from build123d import *

# Parameters (mm, degrees)
F0_W     = 45
F0_H     = 10
F0_R     = 3
F0_R_2   = 2
F1_DEPTH = 10
F2_R     = 4
F3_R     = 3
F5_DEPTH = 2


with BuildPart() as f1:
    # F0 (on Top) → F1 (new body)
    with BuildSketch(Plane.XY):
        Rectangle(F0_W, F0_H)
        Circle(F0_R, mode=Mode.SUBTRACT)
        Circle(F0_R)
        Circle(F0_R_2, mode=Mode.SUBTRACT)
    extrude(amount=F1_DEPTH)

    # F2
    f2_edges = [f1.edges().sort_by_distance(p)[0] for p in [
        (-22.5, -5, 5),
        (22.5, -5, 5),
        (22.5, 5, 5),
        (-22.5, 5, 5),
    ]]
    fillet(f2_edges, radius=F2_R)

    # F3
    f3_edges = [f1.edges().sort_by_distance(p)[0] for p in [
        (0, -5, 10),
        (0, 5, 10),
        (21.328427, 3.828427, 10),
        (-21.328427, 3.828427, 10),
        (22.5, 0, 10),
        (-22.5, 0, 10),
        (21.328427, -3.828427, 10),
        (-21.328427, -3.828427, 10),
    ]]
    fillet(f3_edges, radius=F3_R)

    # F4 (on face) → F5 (cut)
    with BuildSketch(Plane.XY.offset(10)):
        with BuildLine():
            ThreePointArc((0, 2), (1.4142135624, 1.4142135624), (2, 0))
            ThreePointArc((2, 0), (1.4142135624, -1.4142135624), (0, -2))
            Line((0, -2), (2.2360679775, -2))
            ThreePointArc((2.2360679775, -2), (2.8025170769, -1.0704662693), (3, 0))
            ThreePointArc((3, 0), (2.8025170769, 1.0704662693), (2.2360679775, 2))
            Line((2.2360679775, 2), (0, 2))
        make_face()
        with BuildLine():
            Line((-2.2360679775, 2), (0, 2))
            Line((0, 2), (2.2360679775, 2))
            ThreePointArc((2.2360679775, 2), (0, 3), (-2.2360679775, 2))
        make_face()
        with BuildLine():
            ThreePointArc((0, -2), (-2, 0), (0, 2))
            Line((0, 2), (-2.2360679775, 2))
            ThreePointArc((-2.2360679775, 2), (-3, 0), (-2.2360679775, -2))
            Line((-2.2360679775, -2), (0, -2))
        make_face()
        with BuildLine():
            Line((2.2360679775, -2), (0, -2))
            Line((0, -2), (-2.2360679775, -2))
            ThreePointArc((-2.2360679775, -2), (0, -3), (2.2360679775, -2))
        make_face()
    extrude(amount=-F5_DEPTH, mode=Mode.SUBTRACT)


solid = f1.part
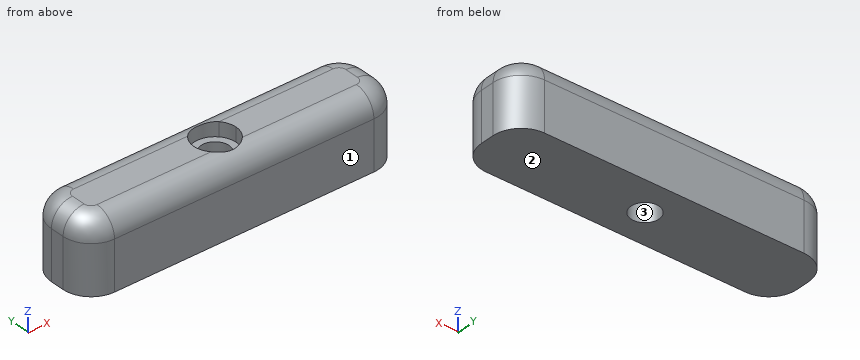
The listing builds one solid part. Answer for the finished solid, in the listing's coordinates (mm). Face numbers are marked on the shaded views. Coordinates: 2 decimals unless noted, no trailing zeros. Write each loop counter-clockwise with the first axis right and the second up, starting at its lowest first coordinate (ties: lowest second). Pieces come first, ordered by that corner, then holes. Notation, with made-up numbers: M -19.75,58 L 11.25,58 A17 cw 11.25,72 Z; hole C 11,10.5 d3. An arc over 180 degrees is marked long. Put each result on its own line as item: value. Start each with the question number.
1. A cutting plane is placed at A-A on z = 5.75. Write down the section's boundary in (x, y).
2. Consider line 1 (Y direction, x = 0, z = 4.75); line 2 (X direction, y = 0, z = 6); line 3 (X direction, y = 0, z = 8.65). Determine where each line is inside the solid, lowest interval first. Write a range as from..to.
3. A cutting plane is placed at B-B on x = 0. Write down the section's boundary in (y, z).
4. For a pull along Y with two mould halves and no side action, classify the marked faces 1, 2 and 3 as pulls with the +Y half, pulls with the -Y half, needs draft (parallel to the pull), parting line crosses it, or undercut.
5. A flat-ended cylindrical pin translates along its axis: P1, Ø3, axis at x = -0.5, y = -1, coming from the +Z side. Find the tip coordinate at first contact, or state that the pin passes through.
6. A cutting plane is placed at C-C on x = -8. Write down the section's boundary in (y, z), then the cut area to 3 significant figures.
Resolved:
1. outline: M -22.5,-1 A4 ccw -18.5,-5 L 18.5,-5 A4 ccw 22.5,-1 L 22.5,1 A4 ccw 18.5,5 L -18.5,5 A4 ccw -22.5,1 Z; hole C 0,0 d4
2. line 1: y = -5..-2, 2..5
2. line 2: x = -22.5..-2, 2..22.5
2. line 3: x = -22.01..-3, 3..22.01
3. outline: M -5,0 L -2,0 L -2,8 L -3,8 L -3,9.83 A3 ccw -5,7 Z; M 2,0 L 5,0 L 5,7 A3 ccw 3,9.83 L 3,8 L 2,8 Z
4. face 1: pulls with the -Y half
4. face 2: needs draft
4. face 3: undercut
5. P1: stops at z = 8
6. outline: M -5,0 L 5,0 L 5,7 A3 ccw 2,10 L -2,10 A3 ccw -5,7 Z
6. area: 96.1 mm2
